Verification items for the finished model (mm, model axes). Face numbers are marked on the shaded views. A direction names the side the tool comes from. Give positions to 0.01 mm unless a question says otherwise; leave off trailing zeros. Order: outer loops, then holes, each group sorted by start corner. A loop starts at its lowest first (then second) coordinate and runs counter-clockwise, first axis right, second up. Notation, with made-up numbers: (-18, -19) -> (22, -19) arc R15 cw to (22, -15) -> close; hole circle Ø8 at (-18.75, 27.5). An arc over 180 degrees is marked (long way). One line per question, with ' | ' between items. Start each with the question number.
Q1. Section check A-A on y = -6.7. Record the cut outline in (x, z), plus the area to 3 significant figures.
Q2. Material ranges on probe 1 along Y at (x, z) = (31, -0.35); probe 2 along Z at (x, y) = (-26, 5.25); probe 3 along Z at (x, y) = (-10.5, -3.25), recorded low to high. Write a range as [from, to].
Q3. Go/stop test with flat-tipped pins: pin 1 (6.5 mm diameter, centred on x = -22.5, y = 7.5, fed in from -Z); pin 2 (8.5 mm diameter, centred on x = -31, y = -6.7, fed in from +Z); pin 3 (1.1 mm diameter, centred on x = -29.5, z = -0.5, fed in from +Y); pin 4 (1.5 mm diameter, centred on y = -7.5, z = 2.5, fed in from -X). Record where each tip stops, or that it passes through.
Q4. Mould release check, pull along X, two halves, no side actions. Record for the marked faces 1, 2, 3 and 4: released by +X, released by -X, zero draft, split by the parting line, or undercut.
Q5. Access from +Z, -Z, +X, -X, +Y, -Y to the whole of each face (thin tool, end or side, straight path). Record for the marked faces 5, 6 and 7.
Q6. Section check B-B on x = -15. Record the cut outline in (y, z).
Q7. Section check C-C on y = 7.25. Record the cut outline in (x, z).
Q8. Section check D-D on x = -31. Record the cut outline in (y, z), plus the area to 3 significant figures.
from build123d import *

# Parameters (mm, degrees)
SKETCH1_W           = 76
SKETCH1_H           = 20
BASE_FLANGE1_DEPTH  = 1
SKETCH6_R           = 2.6
CUT_EXTRUDE1_DEPTH  = 10
SKETCH7_W           = 30
SKETCH7_H           = 10
CUT_EXTRUDE2_DEPTH  = 10
BOSS_EXTRUDE1_DEPTH = 8


# Sheet-metal steps are written as plain solids
with BuildPart() as part:
    # Sketch1 → Base-Flange1 (new body)
    with BuildSketch(Plane.XY):
        Rectangle(SKETCH1_W, SKETCH1_H)
    extrude(amount=-BASE_FLANGE1_DEPTH)

    # Sketch6 → Cut-Extrude1 (cut)
    with BuildSketch(Plane.XY):
        with Locations((-31, -6.7)):
            Circle(SKETCH6_R)
        with Locations(Location((31, -6.7, 0), (0, 0, 180))):
            Circle(SKETCH6_R)
    extrude(amount=-CUT_EXTRUDE1_DEPTH, mode=Mode.SUBTRACT)

    # Sketch7 → Cut-Extrude2 (cut)
    with BuildSketch(Plane.XY):
        with Locations((-23, 5)):
            Rectangle(SKETCH7_W, SKETCH7_H)
        with Locations((23, 5)):
            Rectangle(SKETCH7_W, SKETCH7_H)
    extrude(amount=-CUT_EXTRUDE2_DEPTH, mode=Mode.SUBTRACT)

    # Sketch8 → Boss-Extrude1 (add)
    with BuildSketch(Plane(origin=(0, 10, 0), x_dir=(1, 0, 0), z_dir=(0, 1, 0))):
        Polygon((8, 0), (11.67711212, -3.67711212), (29.020618382, -3.67711212), (33.697730502, 1), (32.28351694, 1), (28.60640482, -2.67711212), (12.091325682, -2.67711212), (8.414213562, 1), (8, 1), align=None)
        Polygon((-32.28351694, 1), (-33.697730502, 1), (-29.020618382, -3.67711212), (-11.67711212, -3.67711212), (-8, 0), (-8, 1), (-8.414213562, 1), (-12.091325682, -2.67711212), (-28.60640482, -2.67711212), align=None)
    extrude(amount=-BOSS_EXTRUDE1_DEPTH)


solid = part.part
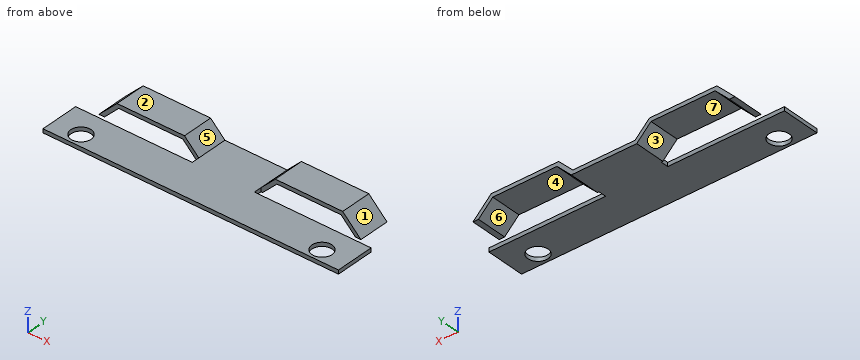
Filled in:
1) outline: (-38, -1) -> (-33.6, -1) -> (-33.6, 0) -> (-38, 0) -> close; (-28.4, -1) -> (28.4, -1) -> (28.4, 0) -> (-28.4, 0) -> close; (33.6, -1) -> (38, -1) -> (38, 0) -> (33.6, 0) -> close | area: 65.6 mm²
2) probe 1: [-10, -9.3], [-4.1, 0] | probe 2: [2.68, 3.68] | probe 3: [-1, 0]
3) pin 1: z = 2.68 | pin 2: z = 0 | pin 3: y = 0 | pin 4: through
4) face 1: released by +X | face 2: zero draft | face 3: undercut | face 4: undercut
5) face 5: +Z, +Y, -Y | face 6: -Z, +Y | face 7: -Z, +Y, -Y
6) outline: (-10, -1) -> (0, -1) -> (0, 0) -> (-10, 0) -> close; (2, 2.68) -> (10, 2.68) -> (10, 3.68) -> (2, 3.68) -> close
7) outline: (-33.7, -1) -> (-32.28, -1) -> (-28.61, 2.68) -> (-12.09, 2.68) -> (-8.41, -1) -> (8.41, -1) -> (12.09, 2.68) -> (28.61, 2.68) -> (32.28, -1) -> (33.7, -1) -> (29.02, 3.68) -> (11.68, 3.68) -> (8, 0) -> (-8, 0) -> (-11.68, 3.68) -> (-29.02, 3.68) -> close
8) outline: (-10, -1) -> (-9.3, -1) -> (-9.3, 0) -> (-10, 0) -> close; (-4.1, -1) -> (0, -1) -> (0, 0) -> (-4.1, 0) -> close; (2, 0.28) -> (10, 0.28) -> (10, 1.7) -> (2, 1.7) -> close | area: 16.1 mm²
